```python
from build123d import *

# Parameters (mm, degrees)
BOSS_EXTRUDE1_DEPTH    = 76.2
CUT_EXTRUDE1_DEPTH     = 118.745
CUT_EXTRUDE2_START     = -12.7
CUT_EXTRUDE2_OUTLINE_W = 8.255
CUT_EXTRUDE2_OUTLINE_H = 30.7975
CUT_EXTRUDE2_DEPTH     = 12.7
SIDECUT_DEPTH          = 166.55395044


# Read off the part's stored shape, not the designer's step: Cut-Extrude2
with BuildPart() as part:
    # Sketch8 → Boss-Extrude1 (new body)
    with BuildSketch(Plane(origin=(0, 0, 0), x_dir=(1, 0, 0), z_dir=(0, 1, 0))):
        Polygon((-73.9775, 8.255), (-73.9775, 0), (73.9775, 0), (73.9775, 8.255), (69.215, 8.255), (69.215, 127), (60.96, 127), (60.96, 8.255), (-60.96, 8.255), (-60.96, 127), (-69.215, 127), (-69.215, 8.255), align=None)
    extrude(amount=BOSS_EXTRUDE1_DEPTH)

    # Sketch9 → Cut-Extrude1 (cut)
    with BuildSketch(Plane(origin=(0, 0, -127), x_dir=(-1, 0, 0), z_dir=(0, 0, -1))):
        Polygon((-66.421, 0), (-66.675, 12.697459746), (-63.5, 12.697459746), (-63.754, 0), align=None)
        Polygon((63.5, 12.697459746), (63.754, 0), (66.421, 0), (66.675, 12.697459746), align=None)
    extrude(amount=-CUT_EXTRUDE1_DEPTH, mode=Mode.SUBTRACT)

    # Cut-Extrude2 outline → Cut-Extrude2 (cut)
    with BuildSketch(Plane.XZ.offset(CUT_EXTRUDE2_START)):
        with Locations((65.0875, -42.70375)):
            Rectangle(CUT_EXTRUDE2_OUTLINE_W, CUT_EXTRUDE2_OUTLINE_H)
        with Locations((65.0875, -92.55125)):
            Rectangle(CUT_EXTRUDE2_OUTLINE_W, CUT_EXTRUDE2_OUTLINE_H)
        Polygon((62.9285, -8.255), (73.9775, -8.255), (73.9775, 0), (62.9285, 0), (62.9285, -2.54), (26.9875, -2.54), (26.9875, 0), (-26.9875, 0), (-26.9875, -2.54), (-62.9285, -2.54), (-62.9285, 0), (-73.9775, 0), (-73.9775, -8.255), (-62.9285, -8.255), (-62.9285, -5.715), (-26.9875, -5.715), (-26.9875, -8.255), (26.9875, -8.255), (26.9875, -5.715), (62.9285, -5.715), align=None)
        with Locations((-65.0875, -42.70375)):
            Rectangle(CUT_EXTRUDE2_OUTLINE_W, CUT_EXTRUDE2_OUTLINE_H)
        with Locations((-65.0875, -92.55125)):
            Rectangle(CUT_EXTRUDE2_OUTLINE_W, CUT_EXTRUDE2_OUTLINE_H)
    extrude(amount=CUT_EXTRUDE2_DEPTH, mode=Mode.SUBTRACT)

    # Sketch8<6> → SideCut (cut, through all)
    with BuildSketch(Plane(origin=(0, 0, 0), x_dir=(1, 0, 0), z_dir=(0, 1, 0))):
        with BuildLine():
            Line((-73.9775, 8.255), (-73.9775, 0))
            Line((-73.9775, 0), (73.9775, 0))
            Line((73.9775, 0), (73.9775, 8.255))
            Line((73.9775, 8.255), (69.215, 8.255))
            Line((69.215, 8.255), (69.215, 127))
            Line((69.215, 127), (60.96, 127))
            Line((60.96, 127), (60.96, 8.255))
            Line((60.96, 8.255), (-63.5, 8.255))
            Line((-63.5, 8.255), (-63.5, 5.902378957))
            ThreePointArc((-63.5, 5.902378957), (-65.0875, 1.74625), (-66.675, 5.902378957))
            Line((-66.675, 5.902378957), (-66.675, 8.255))
            Line((-66.675, 8.255), (-73.9775, 8.255))
        make_face()
    extrude(amount=SIDECUT_DEPTH, mode=Mode.SUBTRACT)


solid = part.part
```
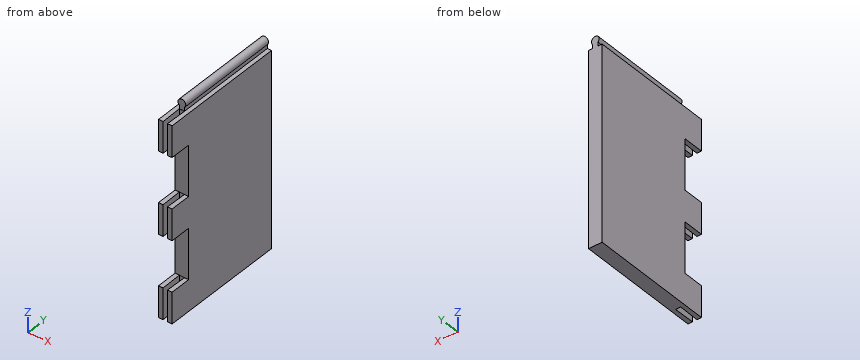
Part model, mm, in its own coordinate system. Coordinates: 2 decimals unless noted, no trailing zeros. Write each loop counter-clockwise with the first axis right and the second up, starting at its lowest first coordinate (ties: lowest second). Pieces come first, ordered by that corner, then holes.
Item 1: Slice it at A-A (z = -117). Write the cut outline in (x, y) (3 decimals).
Item 2: Slice it at C-C (z = -50). Write the cut outline in (x, y) (3 decimals).
Item 3: Pin check, flat tips, straight feed: pin 1 (1.6 mm diameter, centred on x = -65.5, z = -119, fed in from -Y); pin 2 (4 mm diameter, centred on x = -66, y = 7.5, fed in from +Z) (3 decimals); pin 3 (2.5 mm diameter, centred on y = 49, z = -6.5, fed in from -X). Stop position of each tip, or through.
Item 4: Slice it at B-B (y = 33). Write the cut outline in (x, z) (1 decimal), and give its area (3 significant figures).
Item 5: Probe line 1 (Z direction, x = -61.25, y = 70) (3 decimals); line 2 (Y direction, x = -61.5, z = -56); line 3 (Z direction, x = -67.25, y = 46) (3 decimals). List the from-to ranges inside material, lowest first.
Results found:
1. outline: (-69.215, 0) - (-66.421, 0) - (-66.675, 12.697) - (-63.5, 12.697) - (-63.754, 0) - (-60.96, 0) - (-60.96, 76.2) - (-69.215, 76.2) - close
2. outline: (-69.215, 12.7) - (-60.96, 12.7) - (-60.96, 76.2) - (-69.215, 76.2) - close
3. pin 1: stops at y = 12.7
3. pin 2: stops at z = -8.255
3. pin 3: stops at x = -67.19
4. outline: (-69.2, -127) - (-61, -127) - (-61, -8.3) - (-63.5, -8.3) - (-63.5, -5.9) arc R2.4 ccw (long way) to (-66.7, -5.9) - (-66.7, -8.3) - (-69.2, -8.3) - close
4. area: 1,000 mm2
5. line 1: z = -127 to -8.255
5. line 2: y = 12.7 to 76.2
5. line 3: z = -127 to -8.255, -5.124 to -3.131
